Here's how the part is built. I have some questions about the finished solid (model axes, mm). A direction names the side the tool comes from. Give positions to 0.01 mm unless a question says otherwise; leave off trailing zeros. Write each loop counter-clockwise with the first axis right and the second up, starting at its lowest first coordinate (ties: lowest second). Pieces come first, ordered by that corner, then holes. Notation, with made-up numbers: (-39.75, 65.5) - (-23.75, 65.5) arc R27 cw to (-23.75, 83.5) - close; hole circle Ø8 at (79, 26.25). An arc over 180 degrees is marked (long way). Use a Markdown table: item, result.
```python
from build123d import *

# Parameters (mm, degrees)
SKETCH2_R           = 1.1
SKETCH2_R_2         = 4.5
BOSS_EXTRUDE1_DEPTH = 3.048


with BuildPart() as part:
    # Sketch2 → Boss-Extrude1 (new body)
    with BuildSketch(Plane(origin=(0, 0, 0), x_dir=(1, 0, 0), z_dir=(0, 1, 0))):
        with BuildLine():
            Line((28.5, -66.94), (28.5, -32.09))
            ThreePointArc((28.5, -32.09), (28.939339828, -31.029339828), (30, -30.59))
            Line((30, -30.59), (84.83, -30.59))
            ThreePointArc((84.83, -30.59), (85.890660172, -30.150660172), (86.33, -29.09))
            Line((86.33, -29.09), (86.33, -14.88))
            ThreePointArc((86.33, -14.88), (81.971748904, -4.358251096), (71.45, 0))
            Line((71.45, 0), (3, 0))
            ThreePointArc((3, 0), (0.878679656, -0.878679656), (0, -3))
            Line((0, -3), (0, -70.84))
            ThreePointArc((0, -70.84), (0.878679656, -72.961320344), (3, -73.84))
            Line((3, -73.84), (83.340051803, -73.84))
            ThreePointArc((83.340051803, -73.84), (85.333792006, -73.081651177), (86.319565186, -71.19))
            ThreePointArc((86.319565186, -71.19), (85.361009601, -69.232059783), (83.33, -68.44))
            Line((83.33, -68.44), (30, -68.44))
            ThreePointArc((30, -68.44), (28.939339828, -68.000660172), (28.5, -66.94))
        make_face()
        with Locations(Location((4.19, -71.01, 0), (0, 0, 90))):
            Circle(SKETCH2_R, mode=Mode.SUBTRACT)
        with Locations(Location((25.03, -71.01, 0), (0, 0, 90))):
            Circle(SKETCH2_R, mode=Mode.SUBTRACT)
        with Locations(Location((4.19, -2.98, 0), (0, 0, 90))):
            Circle(SKETCH2_R, mode=Mode.SUBTRACT)
        with Locations(Location((51.82, -2.98, 0), (0, 0, 90))):
            Circle(SKETCH2_R, mode=Mode.SUBTRACT)
        with Locations(Location((51.82, -26.2, 0), (0, 0, 90))):
            Circle(SKETCH2_R, mode=Mode.SUBTRACT)
        with Locations(Location((82.13, -71.01, 0), (0, 0, 90))):
            Circle(SKETCH2_R, mode=Mode.SUBTRACT)
        with Locations(Location((82.13, -26.2, 0), (0, 0, 90))):
            Circle(SKETCH2_R, mode=Mode.SUBTRACT)
        with Locations(Location((71.83, -14.33, 0), (0, 0, 90))):
            Circle(SKETCH2_R_2, mode=Mode.SUBTRACT)
        with BuildLine():
            Line((6.5, -6.84), (6.5, -57.34))
            ThreePointArc((6.5, -57.34), (6.353553391, -57.693553391), (6, -57.84))
            Line((6, -57.84), (3.5, -57.84))
            ThreePointArc((3.5, -57.84), (3.146446609, -57.693553391), (3, -57.34))
            Line((3, -57.34), (3, -6.84))
            ThreePointArc((3, -6.84), (3.146446609, -6.486446609), (3.5, -6.34))
            Line((3.5, -6.34), (6, -6.34))
            ThreePointArc((6, -6.34), (6.353553391, -6.486446609), (6.5, -6.84))
        make_face(mode=Mode.SUBTRACT)
        with BuildLine():
            Line((24.5, -6.84), (24.5, -57.34))
            ThreePointArc((24.5, -57.34), (24.353553391, -57.693553391), (24, -57.84))
            Line((24, -57.84), (21.5, -57.84))
            ThreePointArc((21.5, -57.84), (21.146446609, -57.693553391), (21, -57.34))
            Line((21, -57.34), (21, -6.84))
            ThreePointArc((21, -6.84), (21.146446609, -6.486446609), (21.5, -6.34))
            Line((21.5, -6.34), (24, -6.34))
            ThreePointArc((24, -6.34), (24.353553391, -6.486446609), (24.5, -6.84))
        make_face(mode=Mode.SUBTRACT)
    extrude(amount=BOSS_EXTRUDE1_DEPTH)


solid = part.part
```
Item 1: If we section it at C-C, the plane x = 82.13: Write out the boundary of the cut face in (y, z).
Values:
| item | result |
|---|---|
| outline | (0, 4.52) - (3.05, 4.52) - (3.05, 25.1) - (0, 25.1) - close; (0, 27.3) - (3.05, 27.3) - (3.05, 30.59) - (0, 30.59) - close; (0, 68.44) - (3.05, 68.44) - (3.05, 69.91) - (0, 69.91) - close; (0, 72.11) - (3.05, 72.11) - (3.05, 73.84) - (0, 73.84) - close |
Item 2: For faces 1 (the flat face through (43, 2, 73.84)), 2 (the flat face through (5, 2, 6.34)), 3 (the flat face through (28.5, 2, 50)), which set-ups out of +Z, -Z, +X, -X, +Y, -Y let a thin tool reach every point of the face, with its end or its side?
Values:
| item | result |
|---|---|
| face 1 | +Z, +X, -X, +Y, -Y |
| face 2 | +Y, -Y |
| face 3 | +X, +Y, -Y |
Item 3: Will this pin go through, and if not, where does the flat tip stop? pin 1 Ø1.5 at (y, z) = (2, 52.5) entering from +X.
Values:
| item | result |
|---|---|
| pin 1 | stops at x = 28.5 |
Item 4: I need wall thicknesses on line 1 along Z through (x, y) = (51.82, 1.25); line 2 along X through (y, z) = (1.7, 22); line 3 along X through (y, z) = (1.65, 14.33). Which ranges of each line are inside material? Lowest first, please. Write a range as [from, to].
Values:
| item | result |
|---|---|
| line 1 | z = [0, 1.88], [4.08, 25.1], [27.3, 30.59], [68.44, 73.84] |
| line 2 | x = [0, 3], [6.5, 21], [24.5, 86.33] |
| line 3 | x = [0, 3], [6.5, 21], [24.5, 67.33], [76.33, 86.32] |
Item 5: If we section it at D-D, the plane z = 24: Write out the boundary of the cut face in (x, y).
Values:
| item | result |
|---|---|
| outline | (0, 0) - (3, 0) - (3, 3.05) - (0, 3.05) - close; (6.5, 0) - (21, 0) - (21, 3.05) - (6.5, 3.05) - close; (24.5, 0) - (86.33, 0) - (86.33, 3.05) - (24.5, 3.05) - close |
Item 6: Thinking about a two-plate mould opening in X: for faces 4 (the cylindrical face through (3.1, 1.5, 3.12)), 5 (the cylindrical face through (82.087, 1.503, 4.475)), 6 (the cylindrical face through (50.73, 1.5, 26.34)), 7 (the flat face through (57, 2, 30.59)), which applies, +X half, -X half, draft (parallel to the pull), parting line (faces both ways), or undercut?
Values:
| item | result |
|---|---|
| face 4 | undercut |
| face 5 | +X half |
| face 6 | undercut |
| face 7 | draft |
Item 7: If we section it at A-A, the plane x = 33: Write out the boundary of the cut face in (y, z), plus the area to 3 significant figures.
Values:
| item | result |
|---|---|
| outline | (0, 0) - (3.05, 0) - (3.05, 30.59) - (0, 30.59) - close; (0, 68.44) - (3.05, 68.44) - (3.05, 73.84) - (0, 73.84) - close |
| area | 110 mm2 |
Item 8: If we section it at B-B, the plane z = 33: Write out the boundary of the cut face in (x, y), plus the area to 3 significant figures.
Values:
| item | result |
|---|---|
| outline | (0, 0) - (3, 0) - (3, 3.05) - (0, 3.05) - close; (6.5, 0) - (21, 0) - (21, 3.05) - (6.5, 3.05) - close; (24.5, 0) - (28.5, 0) - (28.5, 3.05) - (24.5, 3.05) - close |
| area | 65.5 mm2 |
